Could you check a few things on this model? Use its own coordinates, in mm. A direction names the side the tool comes from. Coordinates: 2 decimals unless noted, no trailing zeros. Write each loop counter-clockwise with the first axis right and the second up, starting at its lowest first coordinate (ties: lowest second). Pieces come first, ordered by that corner, then holes.
```python
from build123d import *

# Parameters (mm, degrees)
SKETCH2_R               = 6
BOSS_EXTRUDE2_DEPTH     = 1
FILLET1_R               = 1
SKETCH3_R               = 2.5
SKETCH3_R_2             = 2
CUT_EXTRUDE1_DEPTH      = 1
BOSS_EXTRUDE3_START     = -3.5
BOSS_EXTRUDE3_OUTLINE_R = 1.5
BOSS_EXTRUDE3_DEPTH     = 2.5
FILLET2_R               = 0.25
FILLET3_R               = 0.25
CHAMFER1_SIZE           = 1.036815955
CHAMFER1_SIZE_2         = 1


# Read off the part's stored shape, not the designer's step: Boss-Extrude1, Boss-Extrude3
# Some blends are built 0.0001 mm under size
with BuildPart() as part:
    # Boss-Extrude1 outline → Boss-Extrude1 (revolve)
    with BuildSketch(Plane.XY):
        Polygon((5, 0), (4.790475383, 6), (0, 6), (0, 0), align=None)
    revolve(axis=Axis((0, 0, 0), (0, 1, 0)))

    # Sketch2 (on Top Plane) → Boss-Extrude2 (add)
    with BuildSketch(Plane(origin=(0, 0, 0), x_dir=(1, 0, 0), z_dir=(0, 1, 0))):
        with Locations(Location((0, 0, 0), (0, 0, 90))):
            Circle(SKETCH2_R)
    extrude(amount=-BOSS_EXTRUDE2_DEPTH)

    # Fillet1
    fillet1_edges = [part.edges().sort_by_distance(p)[0] for p in [
        (-4.790475383, 6, 0),
    ]]
    fillet(fillet1_edges, radius=FILLET1_R)

    # Sketch3 (on Top Plane) → Cut-Extrude1 (cut)
    with BuildSketch(Plane(origin=(0, 0, 0), x_dir=(1, 0, 0), z_dir=(0, 1, 0))):
        with Locations(Location((0, 0, 0), (0, 0, 90))):
            Circle(SKETCH3_R)
        with Locations(Location((0, 0, 0), (0, 0, 90))):
            Circle(SKETCH3_R_2, mode=Mode.SUBTRACT)
    extrude(amount=-CUT_EXTRUDE1_DEPTH, mode=Mode.SUBTRACT)

    # Boss-Extrude3 outline → Boss-Extrude3 (add)
    with BuildSketch(Plane(origin=(0, 0, 0), x_dir=(1, 0, 0), z_dir=(0, 1, 0)).offset(BOSS_EXTRUDE3_START)):
        Circle(BOSS_EXTRUDE3_OUTLINE_R)
    extrude(amount=BOSS_EXTRUDE3_DEPTH)

    # Fillet2
    fillet2_edges = [part.edges().sort_by_distance(p)[0] for p in [
        (0, -1, 2.5),
        (0, -1, 2),
        (-1.5, -1, 0),
    ]]
    fillet(fillet2_edges, radius=FILLET2_R - 0.0001)  # a hair under: the kernel refuses the full size

    # Fillet3
    fillet3_edges = [part.edges().sort_by_distance(p)[0] for p in [
        (-1.5, -3.5, 0),
    ]]
    fillet(fillet3_edges, radius=FILLET3_R)

    # Chamfer1
    # the kernel refuses this chamfer: 1.036815955, 1 mm, written as the material it adds along each edge
    with BuildSketch(Plane(origin=(0, 0, 0), x_dir=(1, 0, 0), z_dir=(0, 0, 1))) as chamfer1_piece_1_section:
        Polygon((5 + CHAMFER1_SIZE, 0), (5 - CHAMFER1_SIZE_2 * 0.0348994967107, CHAMFER1_SIZE_2 * 0.999390827019), (5, 0), align=None)
    chamfer1_piece_1 = revolve(axis=Axis((0, 0, 0), (0, 1, 0)), mode=Mode.PRIVATE)
    chamfer1_piece_1 = chamfer1_piece_1 & Plane(origin=(0, 0.511488324, 0), x_dir=(0, 0, -1), z_dir=(0, 1, 0)) * Cylinder(6, 25, mode=Mode.PRIVATE)
    add(chamfer1_piece_1)


solid = part.part
```
Item 1: Will these pins go through, and if not, where does the flat tip stop? pin 1 Ø2 at (x, y) = (3.5, 0.5) entering from -Z; pin 2 Ø1.5 at (y, z) = (3, -4.5) entering from -X; pin 3 Ø5 at (x, y) = (3.5, 2) entering from -Z.
Item 2: I want a section at A-A, the plane y = -0.25. List the corners of the cut face in (x, z) for me.
Item 3: I want a section at D-D, the plane y = 4.5. List the corners of the cut face in (x, z) for me, then the cut area to 3 significant figures.
Item 4: If I drill on line 1 along X through (y, z) = (-0.4, 0); line 2 along Y through (x, z) = (0, 2.25); line 3 along Y through (x, z) = (-3.25, 1), over which ranges is the centre line in solid material (lowest first)?
Item 5: Which directions (+Z, -Z, +X, -X, +Y, -Y) give clear straight access to the entire face, cutting with the end or side of a thin tool? Please do faces 1 (the flat face through (1, -1, -3)), 2 (the conical face through (4.668, 3.045, -1.47)).
Item 6: If we mould it in two halves opening along X, with no side actions, what happens to faces 3 (the flat face through (0, -3.5, 0)), 4 (the cylindrical face through (2.44, -0.37, 0.54)), 5 (the flat face through (-2, 0, 1)), 6 (the cylindrical face through (-1.802, -0.476, -5.723))? For each: released by +X, released by -X, zero draft, split by the parting line, or undercut.
Taken from the geometry:
1. pin 1: stops at z = -5.4
1. pin 2: stops at x = -3.15
1. pin 3: stops at z = -5.67
2. outline: circle Ø12 at (0, 0); circle Ø4 at (0, 0); hole circle Ø5 at (0, 0)
3. outline: circle Ø9.69 at (0, 0)
3. area: 73.7 mm2
4. line 1: x = -6 to -2.5, -2 to 2, 2.5 to 6
4. line 2: y = 0 to 6
4. line 3: y = -1 to 6
5. face 1: -Y
5. face 2: +Y
6. face 3: zero draft
6. face 4: undercut
6. face 5: undercut
6. face 6: split by the parting line
